Work out the finished part from the listing and answer in its coordinate system (mm). A direction names the side the tool comes from. Coordinates: 2 decimals unless noted, no trailing zeros. Order: outer loops, then holes, each group sorted by start corner. A loop starts at its lowest first (then second) coordinate and runs counter-clockwise, first axis right, second up. Notation, with made-up numbers: M -33.75,37.5 L -10.75,37.5 A37 ccw -10.75,76.5 Z; hole C -14,-30.75 d10. An arc over 180 degrees is marked long. Use a Markdown table: item, result.
from build123d import *

# Parameters (mm, degrees)
SKETCH_3_W              = 20
SKETCH_3_H              = 20
SKETCH_3_W_2            = 16.4
SKETCH_3_H_2            = 16.4
EXTRUDE_1_DEPTH         = 300
HOLE_WIZARD_4_2_4_2_1_D = 4.2
HOLE_WIZARD_4_2_4_2_2_D = 4.2
HOLE_WIZARD_4_2_4_2_3_D = 4.2
CUT_EXTRUDE_1_REACH     = 303.33
SKETCH_10_R             = 6
HOLE_WIZARD_4_2_4_2_4_D = 4.2


with BuildPart() as part:
    # 草图3 → 凸台-拉伸1 (new body)
    with BuildSketch(Plane.XY):
        with Locations((10, 10)):
            Rectangle(SKETCH_3_W, SKETCH_3_H)
        with Locations((10, 10)):
            Rectangle(SKETCH_3_W_2, SKETCH_3_H_2, mode=Mode.SUBTRACT)
    extrude(amount=-EXTRUDE_1_DEPTH)

    # Ø4.2 (4.2) 直径孔1 (through all)
    with Locations(Plane(origin=(10, 20, -182.5), x_dir=(0, 0, 1), z_dir=(0, 1, 0))):
        with Locations((0, 0), (-30, 0)):
            hole_wizard_4_2_4_2_1 = Hole(HOLE_WIZARD_4_2_4_2_1_D / 2)

    # 镜向1: Ø4.2 (4.2) 直径孔1 across plane
    add(hole_wizard_4_2_4_2_1.mirror(Plane.XY.offset(-150)), mode=Mode.SUBTRACT)

    # Ø4.2 (4.2) 直径孔2 (through all)
    with Locations(Plane(origin=(0, 10, -35), x_dir=(0, 0, -1), z_dir=(-1, 0, 0))):
        with Locations((0, 0), (30, 0)):
            hole_wizard_4_2_4_2_2 = Hole(HOLE_WIZARD_4_2_4_2_2_D / 2)

    # 镜向2: Ø4.2 (4.2) 直径孔2 across plane
    add(hole_wizard_4_2_4_2_2.mirror(Plane.XY.offset(-150)), mode=Mode.SUBTRACT)

    # Ø4.2 (4.2) 直径孔3 (through all)
    with Locations(Plane(origin=(0, 10, -165), x_dir=(0, 0, -1), z_dir=(-1, 0, 0))):
        with Locations((0, 0), (-30, 0)):
            Hole(HOLE_WIZARD_4_2_4_2_3_D / 2)

    # 草图10 → 切除-拉伸1 (cut, up to next)
    with BuildSketch(Plane(origin=(0, 20, 0), x_dir=(1, 0, 0), z_dir=(0, 1, 0)), mode=Mode.PRIVATE) as cut_extrude_1_sk1:
        with Locations(Location((10, 10, 0), (0, 0, 270))):
            Circle(SKETCH_10_R)
    cut_extrude_1_tool1 = extrude(cut_extrude_1_sk1.sketch, amount=-CUT_EXTRUDE_1_REACH, mode=Mode.PRIVATE) & part.part
    cut_extrude_1 = cut_extrude_1_tool1.solids().sort_by_distance((10, 20, -10))[0]
    add(cut_extrude_1, mode=Mode.SUBTRACT)

    # 镜向3: 切除-拉伸1 across plane
    add(cut_extrude_1.mirror(Plane.XY.offset(-150)), mode=Mode.SUBTRACT)

    # Ø4.2 (4.2) 直径孔4 (through all)
    with Locations(Plane(origin=(10, 0, -10), x_dir=(0, 0, -1), z_dir=(0, -1, 0))):
        with Locations((0, 0), (280, 0)):
            Hole(HOLE_WIZARD_4_2_4_2_4_D / 2)


solid = part.part
(1) Determine the mould class of faces 1 (the flat face through (1.8, 10, -148)), 2 (the flat face through (10, 20, -148)), 3 (the flat face through (0, 10, -148)) for opening direction X: pulls with the +X half, pulls with the -X half, needs draft (parallel to the pull), parting line crosses it, or undercut.
Conclusion:
| item | result |
|---|---|
| face 1 | undercut |
| face 2 | needs draft |
| face 3 | pulls with the -X half |
(2) A cutting plane is placed at A-A (y = 14.75). Determine the outline of the cut face in (x, z).
Conclusion:
| item | result |
|---|---|
| outline | M 0,-300 L 1.8,-300 L 1.8,0 L 0,0 Z; M 18.2,-300 L 20,-300 L 20,0 L 18.2,0 Z |
(3) Given P1, Ø9.5, axis at x = 10, z = -10, coming from the +Y side, flat-ended and moving along its own axis, determine where the tip first touches the part or whether it passes through.
Conclusion:
| item | result |
|---|---|
| P1 | y = 1.8 |
(4) Straight lines are drawn through the part: L1, parallel to X at y = 6.5, z = -277; L2, parallel to X at y = 18.7, z = -182.5. For each, find the intervals that lie inside material, in ascending order.
Conclusion:
| item | result |
|---|---|
| L1 | 0 to 1.8, 18.2 to 20 |
| L2 | 0 to 7.9, 12.1 to 20 |
(5) A cutting plane is placed at B-B (z = -243). Determine the outline of the cut face in (x, y).
Conclusion:
| item | result |
|---|---|
| outline | M 0,0 L 20,0 L 20,20 L 0,20 Z; hole M 1.8,1.8 L 18.2,1.8 L 18.2,18.2 L 1.8,18.2 Z |
(6) Which of the six approach directions +Z, -Z, +X, -X, +Y, -Y give full straight-line access (tool end or side, diameter ignored) to faces 4 (the flat face through (10, 0, -148)), 5 (the cylindrical face through (11.802, 19.113, -295.723)), 6 (the flat face through (18.2, 10, -148))?
Conclusion:
| item | result |
|---|---|
| face 4 | +Z, -Z, +X, -X, -Y |
| face 5 | +Y |
| face 6 | +Z, -Z |
